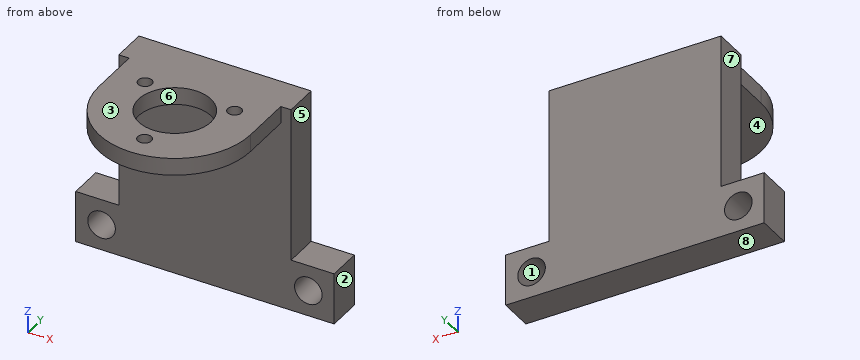
Autodesk Inventor part; units mm, degrees
ref_plane "YZ Plane" through (0, 0, 0) normal (1, 0, 0) x (0, 1, 0)
ref_plane "XZ Plane" through (0, 0, 0) normal (0, 1, 0) x (-1, 0, 0)
ref_plane "XY Plane" through (0, 0, 0) normal (0, 0, 1) x (1, 0, 0)
ref_plane "Work Plane1" through (45.4774, 14.9992, -51) normal (0, 1, 0) x (0, 0, -1)
sketch "Sketch1" plane through (45.4774, 14.9992, -51) normal (0, 1, 0) x (0, 0, -1)
  line L0 (-43.5, 30.4092) -> (-43.5, -29.5908) construction
  line L1 (-36, 37.9092) -> (-51, 37.9092)
  line L2 (-51, 37.9092) -> (-51, -37.0908)
  line L3 (-51, -37.0908) -> (-36, -37.0908)
  line L4 (-36, -37.0908) -> (-36, 37.9092)
  circle A0 centre (-43.5, 30.4092) radius 4
  circle A1 centre (-43.5, -29.5908) radius 4
  line L5 (-51, 25.4092) -> (-91, 25.4092)
  line L6 (-91, 25.4092) -> (-91, -24.5908)
  line L7 (-91, -24.5908) -> (-51, -24.5908)
  line L8 (-51, -24.5908) -> (-51, 25.4092)
  circle A2 centre (93.5, 21.4092) radius 4
  circle A3 centre (93.5, -20.5908) radius 4
  line L9 (51, -30.5908) -> (51, 31.4092)
  line L10 (51, 31.4092) -> (86, 31.4092)
  line L11 (86, 31.4092) -> (86, -30.5908)
  line L12 (86, -30.5908) -> (51, -30.5908)
  circle A4 centre (-43.5, 30.4092) radius 4
  circle A5 centre (43.5, -29.5908) radius 4
  circle A6 centre (0, -29.5908) radius 4
  circle A7 centre (0, 30.4092) radius 4
  circle A8 centre (43.5, 30.4092) radius 4
  circle A9 centre (-43.5, -29.5908) radius 4
  line L13 (-36, -34.5908) -> (-36, 35.4092)
  line L14 (-36, 35.4092) -> (-8, 35.4092)
  line L15 (-8, 35.4092) -> (-8, -34.5908)
  line L16 (-8, -34.5908) -> (-36, -34.5908)
  line L17 (8, -34.5908) -> (8, 35.4092)
  line L18 (8, 35.4092) -> (36, 35.4092)
  line L19 (36, 35.4092) -> (36, -34.5908)
  line L20 (36, -34.5908) -> (8, -34.5908)
  line L21 (-51, -44.5908) -> (101, -44.5908)
  line L22 (101, -44.5908) -> (101, 45.4092)
  line L23 (101, 45.4092) -> (-51, 45.4092)
  line L24 (-51, 45.4092) -> (-51, -44.5908)
  point P0 (-51, 0.4092)
  point P1 (-36, 0.4092)
  dimension "d0" = 75
  dimension "d1" = 15
  dimension "d2" = 40
  dimension "d3" = 50
  dimension "d14" = 8
extrude "Extrusion1" add sketch "Sketch1" along normal blind 10 contours L4 L3 L2 L1 | L2 L7 L6 L5
sketch "Sketch2" plane through (20.0682, 14.9992, 40) normal (0, 0, 1) x (1, 0, 0)
  line L0 (0, 0) -> (50, 0)
  line L1 (50, 0) -> (50, 10)
  line L2 (0, 10) -> (50, 10)
  line L3 (0, 0) -> (0, 10)
  arc A0 (36, -15) -> (14, -15) centre (25, -15) ccw construction
  arc A1 (3, -15) -> (47, -15) centre (25, -15) ccw
  line L4 (3, -15) -> (3, 0)
  line L5 (47, -15) -> (47, 0)
  circle A2 centre (25, -15) radius 10.5
  circle A3 centre (25, -15) radius 15 construction
  circle A4 centre (25, -30) radius 2
  circle A5 centre (12.0096, -7.5) radius 2
  circle A6 centre (37.9904, -7.5) radius 2
  line L6 (25, -15) -> (25, -30) construction
  line L7 (25, -15) -> (37.9904, -7.5) construction
  line L8 (25, -15) -> (12.0096, -7.5) construction
  point P0 (-20.0682, -14.9992)
  dimension "d6" = 22
  dimension "d7" = 21
  dimension "d8" = 30
  dimension "d9" = 4
  dimension "d10" = 120
  dimension "d11" = 120
extrude "Extrusion2" add sketch "Sketch2" along normal blind 5
properties part number "encoder bracket"
Verification items for the finished model (mm, model axes). Face numbers are marked on the shaded views. A direction names the side the tool comes from. Give positions to 0.01 mm unless a question says otherwise; leave off trailing zeros. Write each loop counter-clockwise with the first axis right and the second up, starting at its lowest first coordinate (ties: lowest second). Pieces come first, ordered by that corner, then holes. Notation, with made-up numbers: M 45.25,60.25 L 85.25,60.25 A5 ccw 85.25,64.25 Z; hole C 42.25,55.25 d1. An arc over 180 degrees is marked long. Write item = value, one per line.
(1) Sectioned sample at D-D (z = 8). Record the cut outline in (x, y).
Found:
outline = M 20.07,15 L 70.07,15 L 70.07,25 L 20.07,25 Z
(2) Draft check along X on the marked faces 1, 2 and 3. Enter one of: released by +X, released by -X, zero draft, split by the parting line, or undercut.
Found:
face_1 = undercut
face_2 = released by +X
face_3 = zero draft
(3) Sectioned sample at A-A (z = -7.5). Record the cut outline in (x, y).
Found:
outline = M 7.57,15 L 11.07,15 L 11.07,25 L 7.57,25 Z; M 19.07,15 L 71.07,15 L 71.07,25 L 19.07,25 Z; M 79.07,15 L 82.57,15 L 82.57,25 L 79.07,25 Z
(4) Access from +Z, -Z, +X, -X, +Y, -Y to the whole of each face (thin tool, end or side, straight path). Record for the marked faces 4, 5, 6, 7 and 8.
Found:
face_4 = -Z, +X, -X, -Y
face_5 = +Z, +X, +Y, -Y
face_6 = +Z, -Z
face_7 = +Z, -X, +Y, -Y
face_8 = -Z, +X, -X, +Y, -Y
(5) Go/stop test with flat-tipped pins: pin 1 Ø13 at (x, z) = (75.07, -7.5) entering from +Y; pin 2 Ø3 at (x, y) = (45.07, -15) entering from -Z; pin 3 Ø8 at (y, z) = (21.5, 26) entering from +X; pin 4 Ø2.5 at (y, z) = (6, 42.5) entering from -X. Record where each tip stops, or that it passes through.
Found:
pin_1 = 25
pin_2 = through
pin_3 = 70.07
pin_4 = 23.07
(6) Sectioned sample at C-C (y = -6.5). Record the cut outline in (x, z).
Found:
outline = M 24.05,40 L 36.82,40 L 36.82,45 L 24.05,45 Z; M 53.32,40 L 66.09,40 L 66.09,45 L 53.32,45 Z
(7) Material ranges on line 1 (X direction, y = 19.5, z = -7.5); line 2 (Y direction, x = 41, z = -7); line 3 (Z direction, x = 66, y = -6), recorded low to high.
Found:
line_1 = 7.57 to 11.07, 19.07 to 71.07, 79.07 to 82.57
line_2 = 15 to 25
line_3 = 40 to 45
(8) Sectioned sample at B-B (x = 36). Record the cut outline in (y, z).
Found:
outline = M -20.04,40 L -5.29,40 L -5.29,45 L -20.04,45 Z; M 5.29,40 L 15,40 L 15,-15 L 25,-15 L 25,45 L 5.29,45 Z
